Autodesk Inventor part; units mm, degrees
ref_plane "YZ Plane" through (0, 0, 0) normal (1, 0, 0) x (0, 1, 0)
ref_plane "XZ Plane" through (0, 0, 0) normal (0, 1, 0) x (-1, 0, 0)
ref_plane "XY Plane" through (0, 0, 0) normal (0, 0, 1) x (1, 0, 0)
sketch "Sketch1" plane through (0, 0, 0) normal (1, 0, 0) x (0, 1, 0)
  circle A0 centre (0, 0) radius 8
  circle A1 centre (0, 0) radius 5
  circle A2 centre (0, 0) radius 6.5
  point P0 (6.5, 0)
  point P1 (0, 6.5)
  point P2 (-6.5, 0)
  point P3 (0, -6.5)
  dimension "d0" = 16
  dimension "d5" = 13
extrude "Extrusion1" add sketch "Sketch1" against normal blind 20 contours A0 | A1 | A2
extrude "Extrusion2" add sketch "Sketch1" along normal blind 20 contours A1
hole "Hole1" at (0, 6.5, 0) at (0, 0, 6.5) at (0, -6.5, 0) at (0, 0, -6.5) direction (-1, 0, 0) diameter 2 end through all
properties part number "suspension2chassiscylindricalshaft"
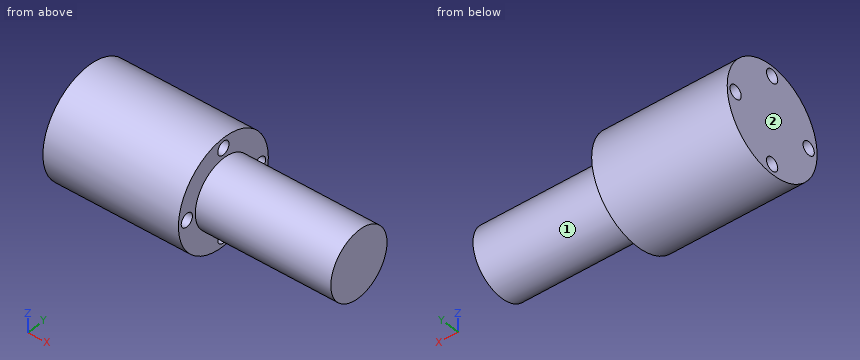
The listing builds one solid part. Answer for the finished solid, in the listing's coordinates (mm). Face numbers are marked on the shaded views. A direction names the side the tool comes from. Give positions to 0.01 mm unless a question says otherwise; leave off trailing zeros. Loops run counter-clockwise (first coordinate to the right, second up) from the corner with the lowest first, then second, coordinate; pieces in that order, holes last. Notation, with made-up numbers: M -25,88 L 21,88 A16 cw 21,92 Z; hole C 12.25,-38 d1. An arc over 180 degrees is marked long. Answer as CSV lines item,"result".
Item 1: Given pin 1 Ø1.6 at (y, z) = (0, 6.5) entering from -X; pin 2 Ø2.5 at (y, z) = (-6.5, 0) entering from +X; pin 3 Ø3 at (x, y) = (-3, -4) entering from -Z; pin 4 Ø2 at (x, z) = (-13, -5) entering from -Y, each flat-ended and moving along its own axis, determine where each tip first touches the part or whether it passes through.
Values follow:
pin 1,"passes through"
pin 2,"stops at x = 0"
pin 3,"stops at z = -7.6"
pin 4,"stops at y = -6.93"
Item 2: The part is cut by section A-A (z = 0). Give the vertices of the cut face in (x, y), and give its area (3 significant figures).
Values follow:
outline,"M -20,-8 L 0,-8 L 0,-7.5 L -20,-7.5 Z; M -20,-5.5 L 0,-5.5 L 0,-5 L 20,-5 L 20,5 L 0,5 L 0,5.5 L -20,5.5 Z; M -20,7.5 L 0,7.5 L 0,8 L -20,8 Z"
area,"440 mm^2"
Item 3: The part is cut by section C-C (z = -6). Give the vertices of the cut face in (x, y), and give its area (3 significant figures).
Values follow:
outline,"M -20,-5.29 L 0,-5.29 L 0,-0.87 L -20,-0.87 Z; M -20,0.87 L 0,0.87 L 0,5.29 L -20,5.29 Z"
area,"177 mm^2"
Item 4: Straight lines are drawn through the part: line 1 along Z through (x, y) = (-11.5, 0); line 2 along Z through (x, y) = (-11.5, 0.75); line 3 along X through (y, z) = (5.5, -1.75). For each, find the intervals that lie inside material, in ascending order. Write a range as [from, to].
Values follow:
line 1,"z = [-8, -7.5], [-5.5, 5.5], [7.5, 8]"
line 2,"z = [-7.96, -7.16], [-5.84, 5.84], [7.16, 7.96]"
line 3,"x = [-20, 0]"
Item 5: The part is cut by section D-D (x = -13). Give the vertices of the cut face in (y, z), and give its area (3 significant figures).
Values follow:
outline,"C 0,0 d16; hole C -6.5,0 d2; hole C 0,-6.5 d2; hole C 0,6.5 d2; hole C 6.5,0 d2"
area,"188 mm^2"
Item 6: Which of the six approach directions +Z, -Z, +X, -X, +Y, -Y give full straight-line access (tool end or side, diameter ignored) to the marked faces 1 and 2?
Values follow:
face 1,"+X"
face 2,"+Z, -Z, -X, +Y, -Y"
